For this review, take the finished solid that the model builds, in its own axes (mm). A direction names the side the tool comes from. Coordinates: 2 decimals unless noted, no trailing zeros. Loops run counter-clockwise (first coordinate to the right, second up) from the corner with the lowest first, then second, coordinate; pieces in that order, holes last. Notation, with made-up numbers: M 12,54 L 45,54 A19 ccw 45,58 Z; hole C -18,5 d9. An arc over 180 degrees is marked long. Answer as a JSON object with one key per item and string values. Group by question number.
Item 1: Mouldability with a two-part tool opening along Y and no side actions: class faces 3 (the face through (61, 58, 13)), 4 (the face through (35, 110, 12)) as +Y half, -Y half, draft (parallel to the pull), parting line (faces both ways), or undercut.
Item 2: Add section B-B (x = 24). State the section outline as (y, z) points, then the cut area to 3 significant figures.
Item 3: Tool access review of faces 1 (the face through (9, 13, 13)), 2 (the face through (61.76, 103.483, 3.326)): name each direction out of +Z, -Z, +X, -X, +Y, -Y from which nothing blocks a thin tool from reaching the whole face with its end or side.
Item 4: Wall thickness on L1, parallel to Y at x = 36, z = 6.5; L2, parallel to X at y = 49, z = 5.25; L3, parallel to Y at x = 61.5, z = 1.5: over which ranges is each line inside the solid? List them lowest first. Write a range as from..to.
Item 5: Add section A-A (y = 91.5). State the section outline as (x, z) points.
Item 6: Add section C-C (z = 9.75). Count the separate pieces of the cut face and the enclosed holes in it, then the cut area to 3 significant figures.
Item 7: Insertion check: pin 1 (9.5 mm diameter, centred on x = 34.5, y = 38, fed in from -Z); pin 2 (2 mm diameter, centred on x = 61.5, y = 101.5, fed in from -Z). Each pin has a flat end and moves straight along its axis. Give the tip position at first contact, or say it passes through.
from build123d import *

# Parameters (mm, degrees)
SKETCH1_W           = 70
SKETCH1_H           = 110
BOSS_EXTRUDE1_DEPTH = 25
SKETCH2_W           = 60.4
SKETCH2_H           = 100.4
CUT_EXTRUDE1_DEPTH  = 1.6
FILLET1_R           = 3
CUT_EXTRUDE4_DEPTH  = 133.467203488
CUT_EXTRUDE5_DEPTH  = 133.467203488
CUT_EXTRUDE6_DEPTH  = 1
SKETCH3_R           = 2
CUT_EXTRUDE7_DEPTH  = 3.5
SKETCH8_W           = 34
SKETCH8_H           = 31
BOSS_EXTRUDE2_DEPTH = 1


with BuildPart() as part:
    # Sketch1 → Boss-Extrude1 (new body)
    with BuildSketch(Plane.XY):
        with Locations((35, 55)):
            Rectangle(SKETCH1_W, SKETCH1_H)
    extrude(amount=BOSS_EXTRUDE1_DEPTH)

    # Sketch2 → Cut-Extrude1 (cut)
    with BuildSketch(Plane(origin=(0, 0, 0), x_dir=(-1, 0, 0), z_dir=(0, 0, -1))):
        with Locations((-35, 55)):
            Rectangle(SKETCH2_W, SKETCH2_H)
    extrude(amount=-CUT_EXTRUDE1_DEPTH, mode=Mode.SUBTRACT)

    # Fillet1
    fillet1_edges = [part.edges().sort_by_distance(p)[0] for p in [
        (65.2, 4.8, 0.8),
        (65.2, 105.2, 0.8),
        (4.8, 105.2, 0.8),
        (4.8, 4.8, 0.8),
    ]]
    fillet(fillet1_edges, radius=FILLET1_R)

    # Sketch5 → Cut-Extrude4 (cut, through all)
    with BuildSketch(Plane(origin=(0, 0, 1.6), x_dir=(-1, 0, 0), z_dir=(0, 0, -1))):
        Polygon((-54, 14), (-16, 14), (-12, 10), (-16, 6), (-54, 6), (-58, 10), align=None)
        Polygon((-58, 55), (-54, 59), (-16, 59), (-12, 55), (-16, 51), (-54, 51), align=None)
        Polygon((-58, 100), (-54, 104), (-16, 104), (-12, 100), (-16, 96), (-54, 96), align=None)
    extrude(amount=-CUT_EXTRUDE4_DEPTH, mode=Mode.SUBTRACT)

    # Sketch6 → Cut-Extrude5 (cut, through all)
    with BuildSketch(Plane(origin=(0, 0, 1.6), x_dir=(-1, 0, 0), z_dir=(0, 0, -1))):
        Polygon((-55, 15), (-55, 50), (-59, 54), (-63, 50), (-63, 15), (-59, 11), align=None)
        Polygon((-15, 50), (-11, 54), (-7, 50), (-7, 15), (-11, 11), (-15, 15), align=None)
        Polygon((-63, 95), (-59, 99), (-55, 95), (-55, 60), (-59, 56), (-63, 60), align=None)
        Polygon((-15, 95), (-11, 99), (-7, 95), (-7, 60), (-11, 56), (-15, 60), align=None)
    extrude(amount=-CUT_EXTRUDE5_DEPTH, mode=Mode.SUBTRACT)

    # Sketch7 → Cut-Extrude6 (cut)
    with BuildSketch(Plane(origin=(0, 0, 1.6), x_dir=(-1, 0, 0), z_dir=(0, 0, -1))):
        Polygon((-55, 95), (-54, 96), (-16, 96), (-15, 95), (-15, 60), (-16, 59), (-54, 59), (-55, 60), align=None)
        Polygon((-54, 14), (-55, 15), (-55, 50), (-54, 51), (-16, 51), (-15, 50), (-15, 15), (-16, 14), align=None)
    extrude(amount=-CUT_EXTRUDE6_DEPTH, mode=Mode.SUBTRACT)

    # Sketch3 → Cut-Extrude7 (cut)
    with BuildSketch(Plane(origin=(0, 0, 1.6), x_dir=(-1, 0, 0), z_dir=(0, 0, -1))):
        with Locations((-61.5, 101.5)):
            Circle(SKETCH3_R)
        with Locations((-61.5, 8.5)):
            Circle(SKETCH3_R)
        with Locations((-8.5, 8.5)):
            Circle(SKETCH3_R)
        with Locations((-8.5, 101.5)):
            Circle(SKETCH3_R)
    extrude(amount=-CUT_EXTRUDE7_DEPTH, mode=Mode.SUBTRACT)

    # Sketch8 → Boss-Extrude2 (add)
    with BuildSketch(Plane(origin=(0, 0, 2.6), x_dir=(-1, 0, 0), z_dir=(0, 0, -1))):
        with Locations((-35, 77.5)):
            Rectangle(SKETCH8_W, SKETCH8_H)
        with Locations((-35, 32.5)):
            Rectangle(SKETCH8_W, SKETCH8_H)
    extrude(amount=BOSS_EXTRUDE2_DEPTH)


solid = part.part
From the geometry:
{
 "1": {"face 3": "undercut", "face 4": "+Y half"},
 "2": {"outline": "M 0,0 L 4.8,0 L 4.8,1.6 L 6,1.6 L 6,25 L 0,25 Z; M 14,2.6 L 17,2.6 L 17,1.6 L 48,1.6 L 48,2.6 L 51,2.6 L 51,25 L 14,25 Z; M 59,2.6 L 62,2.6 L 62,1.6 L 93,1.6 L 93,2.6 L 96,2.6 L 96,25 L 59,25 Z; M 104,1.6 L 105.2,1.6 L 105.2,0 L 110,0 L 110,25 L 104,25 Z", "area": "2,020 mm²"},
 "3": {"face 1": "+Z, -Z", "face 2": "-Z"},
 "4": {"L1": "y = 0..6, 14..51, 59..96, 104..110", "L2": "x = 0..7, 15..55, 63..70", "L3": "y = 0..4.8, 105.2..110"},
 "5": {"outline": "M 0,0 L 4.8,0 L 4.8,1.6 L 7,1.6 L 7,25 L 0,25 Z; M 15,2.6 L 18,2.6 L 18,1.6 L 52,1.6 L 52,2.6 L 55,2.6 L 55,25 L 15,25 Z; M 63,1.6 L 65.2,1.6 L 65.2,0 L 70,0 L 70,25 L 63,25 Z"},
 "6": {"separate pieces": "1", "enclosed holes": "7", "area": "5,440 mm²"},
 "7": {"pin 1": "stops at z = 1.6", "pin 2": "stops at z = 5.1"}
}
